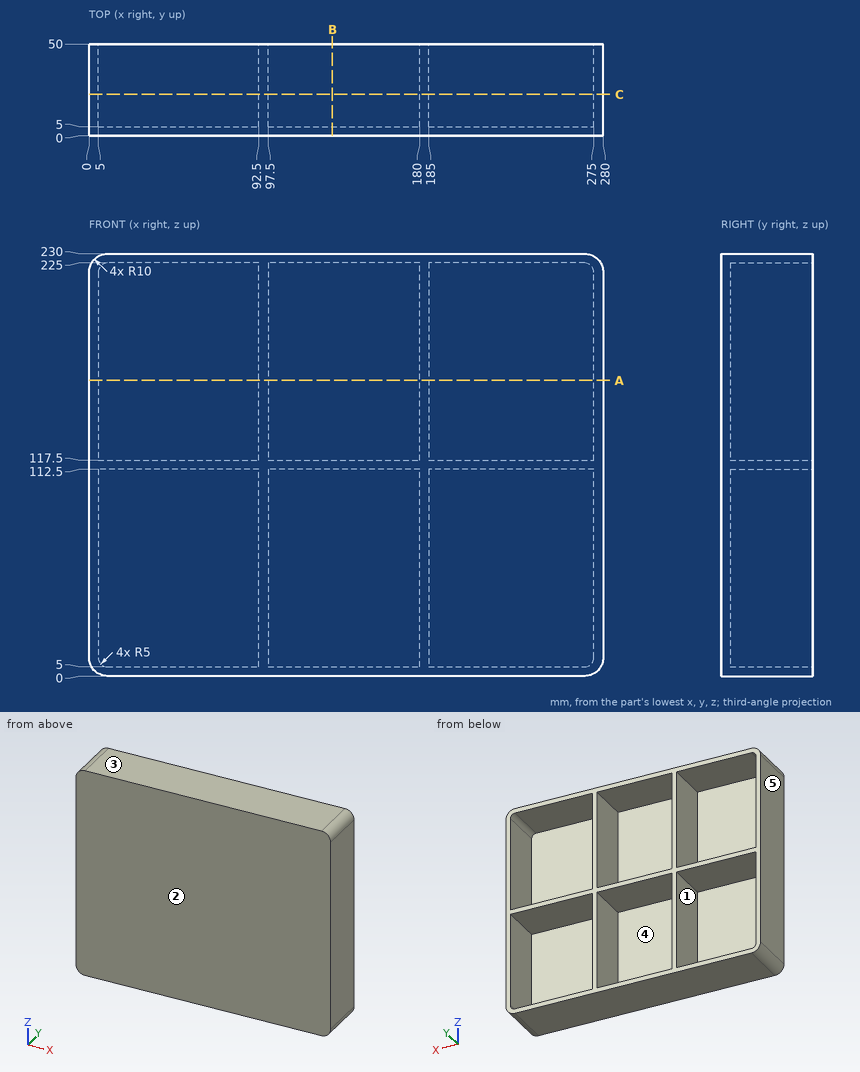
The figure shows three views and two pictorial views of one solid part (mm, origin at its lowest corner). Answer the questions. A direction names the side the tool comes from. Give positions to 0.01 mm unless a question says otherwise; leave off trailing zeros. Write each loop counter-clockwise with the first axis right and the second up, starting at its lowest first coordinate (ties: lowest second). Pieces come first, ordered by that corner, then holes. Notation, with made-up numbers: M -3.5,59 L 14.5,59 A31 ccw 14.5,96 Z; hole C 16,-33 d10. An arc over 180 degrees is marked long. Write each question's results on one line, items separated by ' | '.
Q1. Section A-A, the plane z = 161 is taken. Write down the section's boundary in (x, y), then the cut area to 3 significant figures.
Output values:
outline: M 0,0 L 280,0 L 280,50 L 275,50 L 275,5 L 185,5 L 185,50 L 180,50 L 180,5 L 97.5,5 L 97.5,50 L 92.5,50 L 92.5,5 L 5,5 L 5,50 L 0,50 Z | area: 2,300 mm2
Q2. Section B-B, the plane x = 132.5 is taken. Write down the section's boundary in (y, z).
Output values:
outline: M 0,0 L 50,0 L 50,5 L 5,5 L 5,112.5 L 50,112.5 L 50,117.5 L 5,117.5 L 5,225 L 50,225 L 50,230 L 0,230 Z
Q3. Consider L1, parallel to X at y = 42.5, z = 111; L2, parallel to Z at x = 46.5, y = 26; L3, parallel to Y at x = 76.5, z = 210. Determine where each line is inside the solid, lowest interval first. Write a range as from..to.
Output values:
L1: 0..5, 92.5..97.5, 180..185, 275..280 | L2: 0..5, 112.5..117.5, 225..230 | L3: 0..5
Q4. Section C-C, the plane y = 22.5 is taken. Count the separate pieces of the cut face and the enclosed holes in it, then the cut area to 3 significant figures.
Output values:
separate pieces: 1 | enclosed holes: 6 | area: 8,440 mm2
Q5. A tool of negligible diameter and unlimited length cuts with its end or side. For the marked faces 1 and 2, from which of +Z, -Z, +X, -X, +Y, -Y can it reach the whole face along a straight path? Write none if from no direction.
Output values:
face 1: +Y | face 2: +Z, -Z, +X, -X, -Y
Q6. Flat-ended cylindrical pins translate along their axes: P1, Ø10, axis at x = 179, z = 143, coming from the +Y side; P2, Ø2, axis at x = 87.5, z = 152.5, coming from the +Y side. Find the tip coordinate at first contact, or state that the pin passes through.
Output values:
P1: y = 50 | P2: y = 5
Q7. For a pull along Z with two mould halves and no side action, classify the marked faces 3, 4 and 5 as released by +Z, released by -Z, zero draft, split by the parting line, or undercut.
Output values:
face 3: released by +Z | face 4: undercut | face 5: zero draft
